Geometry: final body of the model. Coordinates: model frame, mm. A direction names the side the tool comes from. Coordinates: 2 decimals unless noted, no trailing zeros. Order: outer loops, then holes, each group sorted by start corner. A loop starts at its lowest first (then second) coordinate and runs counter-clockwise, first axis right, second up. Notation, with made-up numbers: (49.5, -5) -> (106.5, -5) arc R15 cw to (106.5, 24) -> close; hole circle Ø11 at (21.25, 71.25). An arc over 180 degrees is marked (long way). Answer in a Markdown table with one row per item. Add a question column.
1) Set-up query: faces 1 (the face through (-63.5, 15, 1)), 2 (the face through (-113, 15, 12.14)), 3 (the face through (118, 15, 1.86)), 4 (the face through (-5.193, 15, 15)). Return all of +Z, -Z, +X, -X, +Y, -Y with unobstructed straight access to the full face (end or side cutting, diameter ignored); none if empty.
2) Ray query, line 1 (X direction, y = 15.5, z = 4.5); line 2 (Z direction, x = 4.5, y = 15) (3 decimals); line 3 (X direction, y = 16, z = -1). Return the intervals inside material, ascending. Write a range as from..to.
3) Pull-direction query (X, two-part tool) for faces 5 (the face through (-118, 15, -1.38)), 6 (the face through (26.414, 15, -8)); classes: +X half, -X half, draft (parallel to the pull), parting line (faces both ways), or undercut.
4) Section query A-A on x = 76.5. Return the cut outline in (y, z).
5) Section query B-B on z = -8.5. Count the separate pieces of the cut face and the enclosed holes in it, then the cut area to 3 significant figures.
6) Contact query for flat-ended pins moving along their axis: P1, Ø1.8, axis at y = 15, z = -7, coming from the +X side; P2, Ø1.9, axis at x = -10.5, y = 15.5, coming from the -Z side; P3, Ø8, axis at x = 31.5, z = -7, coming from the +Y side; P4, Ø3, axis at y = 15.5, z = 15.5, coming from the -X side. Output: stop coordinate, or through.
```python
from build123d import *

# Parameters (mm, degrees)
PAD006_DEPTH    = 6.3754
SKETCH009_W     = 10.398121
SKETCH009_H     = 6.096
SKETCH009_W_2   = 10.398122
POCKET002_DEPTH = 7.3754
SKETCH011_R     = 3.275
SKETCH011_W     = 13
SKETCH011_H     = 8
POCKET004_DEPTH = 7.3754


with BuildPart() as part:
    # Sketch008 (on DatumPlane) → Pad006 (new body)
    with BuildSketch(Plane.XZ.offset(-11.8547)):
        with BuildLine():
            Line((-110.449725, -30.4013), (-121.115098, -30.4013))
            Line((-121.115098, -30.4013), (-121.115098, -10.9957))
            Line((-121.115098, -10.9957), (-110.449725, -10.9957))
            Line((-110.449725, -10.9957), (-110.449725, -4.8997))
            Line((-110.449725, -4.8997), (-114.739698, -4.8997))
            Line((-114.739698, -4.8997), (-114.739698, -1.38006))
            Line((-114.739698, -1.38006), (-121.115098, -1.38006))
            Line((-121.115098, -1.38006), (-121.115098, 1.86018))
            Line((-121.115098, 1.86018), (-114.739698, 1.86018))
            Line((-114.739698, 1.86018), (-114.739698, 5.37982))
            Line((-114.739698, 5.37982), (-121.115098, 5.37982))
            Line((-121.115098, 5.37982), (-121.115098, 8.62006))
            Line((-121.115098, 8.62006), (-114.739698, 8.62006))
            Line((-114.739698, 8.62006), (-114.739698, 12.1397))
            Line((-114.739698, 12.1397), (-110.449725, 12.1397))
            Line((-110.449725, 12.1397), (-110.449725, 18.5151))
            Line((-110.449725, 18.5151), (-100.063751, 18.5151))
            Line((-100.063751, 18.5151), (-100.063751, 12.1397))
            Line((-100.063751, 12.1397), (-89.398377, 12.1397))
            Line((-89.398377, 12.1397), (-89.398377, 18.5151))
            Line((-89.398377, 18.5151), (-79.012403, 18.5151))
            Line((-79.012403, 18.5151), (-79.012403, 12.1397))
            Line((-79.012403, 12.1397), (-68.34703, 12.1397))
            Line((-68.34703, 12.1397), (-68.34703, 18.5151))
            Line((-68.34703, 18.5151), (-57.961056, 18.5151))
            Line((-57.961056, 18.5151), (-57.961056, 12.1397))
            Line((-57.961056, 12.1397), (-47.295682, 12.1397))
            Line((-47.295682, 12.1397), (-47.295682, 18.5151))
            Line((-47.295682, 18.5151), (-36.909708, 18.5151))
            Line((-36.909708, 18.5151), (-36.909708, 12.1397))
            Line((-36.909708, 12.1397), (-26.244334, 12.1397))
            Line((-26.244334, 12.1397), (-26.244334, 18.5151))
            Line((-26.244334, 18.5151), (-15.858361, 18.5151))
            Line((-15.858361, 18.5151), (-15.858361, 12.1397))
            Line((-15.858361, 12.1397), (-5.192987, 12.1397))
            Line((-5.192987, 12.1397), (-5.192987, 18.5151))
            Line((-5.192987, 18.5151), (5.192987, 18.5151))
            Line((5.192987, 18.5151), (5.192987, 12.1397))
            Line((5.192987, 12.1397), (15.858361, 12.1397))
            Line((15.858361, 12.1397), (15.858361, 18.5151))
            Line((15.858361, 18.5151), (26.244334, 18.5151))
            Line((26.244334, 18.5151), (26.244334, 12.1397))
            Line((26.244334, 12.1397), (36.909708, 12.1397))
            Line((36.909708, 12.1397), (36.909708, 18.5151))
            Line((36.909708, 18.5151), (47.295682, 18.5151))
            Line((47.295682, 18.5151), (47.295682, 12.1397))
            Line((47.295682, 12.1397), (57.961056, 12.1397))
            Line((57.961056, 12.1397), (57.961056, 18.5151))
            Line((57.961056, 18.5151), (68.34703, 18.5151))
            Line((68.34703, 18.5151), (68.34703, 12.1397))
            Line((68.34703, 12.1397), (79.012403, 12.1397))
            Line((79.012403, 12.1397), (79.012403, 18.5151))
            Line((79.012403, 18.5151), (89.398377, 18.5151))
            Line((89.398377, 18.5151), (89.398377, 12.1397))
            Line((89.398377, 12.1397), (100.063751, 12.1397))
            Line((100.063751, 12.1397), (100.063751, 18.5151))
            Line((100.063751, 18.5151), (110.449725, 18.5151))
            Line((110.449725, 18.5151), (110.449725, 12.1397))
            Line((110.449725, 12.1397), (114.739698, 12.1397))
            Line((114.739698, 12.1397), (114.739698, 8.62006))
            Line((114.739698, 8.62006), (121.115098, 8.62006))
            Line((121.115098, 8.62006), (121.115098, 5.37982))
            Line((121.115098, 5.37982), (114.739698, 5.37982))
            Line((114.739698, 5.37982), (114.739698, 1.86018))
            Line((114.739698, 1.86018), (121.115098, 1.86018))
            Line((121.115098, 1.86018), (121.115098, -1.38006))
            Line((121.115098, -1.38006), (114.739698, -1.38006))
            Line((114.739698, -1.38006), (114.739698, -4.8997))
            Line((114.739698, -4.8997), (110.449725, -4.8997))
            Line((110.449725, -4.8997), (110.449725, -10.9957))
            Line((110.449725, -10.9957), (121.115098, -10.9957))
            Line((121.115098, -10.9957), (121.115098, -30.4013))
            Line((121.115098, -30.4013), (110.449725, -30.4013))
            ThreePointArc((110.449725, -30.4013), (108.582413, -25.893211), (104.074325, -24.0259))
            Line((-104.074325, -24.0259), (104.074325, -24.0259))
            ThreePointArc((-104.074325, -24.0259), (-108.582413, -25.893211), (-110.449725, -30.4013))
        make_face()
    extrude(amount=-PAD006_DEPTH)

    # Sketch009 (on Face77 of Pad006) → Pocket002 (cut)
    with BuildSketch(Plane.XZ.offset(-11.8547)):
        with Locations((-94.840395, -7.9477)):
            Rectangle(SKETCH009_W, SKETCH009_H)
        with Locations((-73.764751, -7.9477)):
            Rectangle(SKETCH009_W_2, SKETCH009_H)
        with Locations((-52.689108, -7.9477)):
            Rectangle(SKETCH009_W_2, SKETCH009_H)
        with Locations((-31.613465, -7.9477)):
            Rectangle(SKETCH009_W_2, SKETCH009_H)
        with Locations((-10.537821, -7.9477)):
            Rectangle(SKETCH009_W, SKETCH009_H)
        with Locations((10.537821, -7.9477)):
            Rectangle(SKETCH009_W, SKETCH009_H)
        with Locations((31.613465, -7.9477)):
            Rectangle(SKETCH009_W_2, SKETCH009_H)
        with Locations((52.689108, -7.9477)):
            Rectangle(SKETCH009_W_2, SKETCH009_H)
        with Locations((73.764751, -7.9477)):
            Rectangle(SKETCH009_W_2, SKETCH009_H)
        with Locations((94.840395, -7.9477)):
            Rectangle(SKETCH009_W, SKETCH009_H)
    extrude(amount=-POCKET002_DEPTH, mode=Mode.SUBTRACT)

    # Sketch011 (on Face4 of Pocket002) → Pocket004 (cut)
    with BuildSketch(Plane.XZ.offset(-11.8547)):
        with Locations((4.5, 4.83)):
            Circle(SKETCH011_R)
        with Locations((-56.999992, 1.117064)):
            Rectangle(SKETCH011_W, SKETCH011_H)
    extrude(amount=-POCKET004_DEPTH, mode=Mode.SUBTRACT)


solid = part.part
```
Result:
| question | item | result |
|---|---|---|
| 1 | face 1 | +Y, -Y |
| 1 | face 2 | +Z, -X, +Y, -Y |
| 1 | face 3 | +X, +Y, -Y |
| 1 | face 4 | +Z, +Y, -Y |
| 2 | line 1 | -114.74..-63.5, -50.5..1.24, 7.76..114.74 |
| 2 | line 2 | -24.026..1.555, 8.105..18.515 |
| 2 | line 3 | -121.12..-63.5, -50.5..121.12 |
| 3 | face 5 | draft |
| 3 | face 6 | undercut |
| 4 | outline | (11.85, -24.03) -> (18.23, -24.03) -> (18.23, -11) -> (11.85, -11) -> close; (11.85, -4.9) -> (18.23, -4.9) -> (18.23, 12.14) -> (11.85, 12.14) -> close |
| 5 | separate pieces | 11 |
| 5 | enclosed holes | 0 |
| 5 | area | 745 mm2 |
| 6 | P1 | x = 110.45 |
| 6 | P2 | z = -24.03 |
| 6 | P3 | y = 18.23 |
| 6 | P4 | x = -110.45 |
